from build123d import *

# Parameters (mm, degrees)
SKETCH1_R                                            = 4.5
BOSS_EXTRUDE1_DEPTH                                  = 4
SKETCH2_W                                            = 24
SKETCH2_H                                            = 6
BOSS_EXTRUDE2_DEPTH                                  = 8
CBORE_FOR_M3_HEXAGON_HEAD_BOLTS_FULL_THR_D           = 3.4
CBORE_FOR_M3_HEXAGON_HEAD_BOLTS_FULL_THR_CBORE_D     = 7
CBORE_FOR_M3_HEXAGON_HEAD_BOLTS_FULL_THR_CBORE_DEPTH = 2
FILLET1_R                                            = 10
FILLET2_R                                            = 10
SKETCH4_R                                            = 2.05
SKETCH4_R_2                                          = 1.9812
CUT_EXTRUDE2_DEPTH                                   = 51.635955605


with BuildPart() as part:
    # Sketch1 → Boss-Extrude1 (new body)
    with BuildSketch(Plane(origin=(0, 0, 0), x_dir=(1, 0, 0), z_dir=(0, 1, 0))):
        with BuildLine():
            Line((-16, 0), (-16, -30))
            Line((-16, -30), (16, -30))
            Line((16, -30), (16, 0))
            ThreePointArc((16, 0), (0, 16), (-16, 0))
        make_face()
        with Locations(Location((0, 0, 0), (0, 0, 270))):
            Circle(SKETCH1_R, mode=Mode.SUBTRACT)
    extrude(amount=BOSS_EXTRUDE1_DEPTH)

    # Sketch2 → Boss-Extrude2 (add)
    with BuildSketch(Plane(origin=(0, 4, 0), x_dir=(1, 0, 0), z_dir=(0, 1, 0))):
        with Locations((28, -3)):
            Rectangle(SKETCH2_W, SKETCH2_H)
        with Locations((-28, -3)):
            Rectangle(SKETCH2_W, SKETCH2_H)
    extrude(amount=-BOSS_EXTRUDE2_DEPTH)

    # CBORE for M3 Hexagon head bolts-Full thread-grades AB1 (through all)
    with Locations(Plane(origin=(-35, 0, 6), x_dir=(1, 0, 0), z_dir=(0, 0, 1))):
        with Locations((0, 0), (70, 0)):
            CounterBoreHole(CBORE_FOR_M3_HEXAGON_HEAD_BOLTS_FULL_THR_D / 2, CBORE_FOR_M3_HEXAGON_HEAD_BOLTS_FULL_THR_CBORE_D / 2, CBORE_FOR_M3_HEXAGON_HEAD_BOLTS_FULL_THR_CBORE_DEPTH)

    # Fillet1
    # the kernel refuses this fillet: 10 mm, written as the material it adds along each edge
    with BuildSketch(Plane(origin=(16, 0, 6), x_dir=(-1, 0, 0), z_dir=(0, 0, -1)), Plane(origin=(-16, 0, 0), x_dir=(1, 0, 0), z_dir=(0, 0, 1))) as fillet1_piece_1:
        with BuildLine():
            CenterArc((8, -10), FILLET1_R, 90, 53.130102354)
            Line((0, -4), (0, 0))
            Line((0, 0), (8, 0))
        make_face()
    extrude(amount=6)

    # Fillet2
    fillet2_edges = [part.edges().sort_by_distance(p)[0] for p in [
        (16, -4, 3),
        (-16, -4, 3),
    ]]
    fillet(fillet2_edges, radius=FILLET2_R)

    # Sketch4 → Cut-Extrude2 (cut, through all)
    # profile 1 of 4: a face of its own
    with BuildSketch(Plane(origin=(0, 4, 0), x_dir=(1, 0, 0), z_dir=(0, 1, 0))):
        with Locations(Location((-10.359727729, -15.825724364, 0), (0, 0, 270))):
            Circle(SKETCH4_R)
        with Locations((-10.359727729, -15.825724364)):
            Circle(SKETCH4_R_2, mode=Mode.SUBTRACT)
    # profile 2 of 4: a face of its own
    with BuildSketch(Plane(origin=(0, 4, 0), x_dir=(1, 0, 0), z_dir=(0, 1, 0))):
        with Locations((-10.359727729, -15.825724364)):
            Circle(SKETCH4_R_2)
    # profile 3 of 4: a face of its own
    with BuildSketch(Plane(origin=(0, 4, 0), x_dir=(1, 0, 0), z_dir=(0, 1, 0))):
        with Locations(Location((10.594689167, -15.669399213, 0), (0, 0, 270))):
            Circle(SKETCH4_R)
        with Locations((10.594689167, -15.669399213)):
            Circle(SKETCH4_R_2, mode=Mode.SUBTRACT)
    # profile 4 of 4: a face of its own
    with BuildSketch(Plane(origin=(0, 4, 0), x_dir=(1, 0, 0), z_dir=(0, 1, 0))):
        with Locations((10.594689167, -15.669399213)):
            Circle(SKETCH4_R_2)
    extrude(amount=-CUT_EXTRUDE2_DEPTH, mode=Mode.SUBTRACT)


solid = part.part
Can you work these out from the model? Positions are in its coordinate system, mm. A direction names the side the tool comes from. Coordinates: 2 decimals unless noted, no trailing zeros. Write each loop counter-clockwise with the first axis right and the second up, starting at its lowest first coordinate (ties: lowest second). Pieces come first, ordered by that corner, then holes.
Q1. Imagine slicing it at A-A, the plane x = -35. List the corners of the cut face in (y, z) for me.
Results found:
outline: (-4, 0) - (-1.7, 0) - (-1.7, 4) - (-3.5, 4) - (-3.5, 6) - (-4, 6) - close; (1.7, 0) - (4, 0) - (4, 6) - (3.5, 6) - (3.5, 4) - (1.7, 4) - close
Q2. Imagine slicing it at D-D, the plane z = 8. List the corners of the cut face in (x, y) for me, plus the area to 3 significant figures.
Results found:
outline: (-16, 0) - (16, 0) - (16, 4) - (-16, 4) - close
area: 128 mm2
Q3. Imagine slicing it at C-C, the plane y = 2.75. List the corners of the cut face in (x, z) for me, plus the area to 3 significant figures.
Results found:
outline: (-40, 0) - (-16, 0) arc R16 ccw to (16, 0) - (40, 0) - (40, 6) - (37.17, 6) - (37.17, 4) - (32.83, 4) - (32.83, 6) - (16, 6) - (16, 30) - (-16, 30) - (-16, 6) - (-32.83, 6) - (-32.83, 4) - (-37.17, 4) - (-37.17, 6) - (-40, 6) - close; hole circle Ø4.1 at (-10.36, 15.83); hole circle Ø9 at (0, 0); hole circle Ø4.1 at (10.59, 15.67)
area: 1,540 mm2
Q4. Imagine slicing it at B-B, the plane x = 0. List the corners of the cut face in (y, z) for me.
Results found:
outline: (0, -16) - (4, -16) - (4, -4.5) - (0, -4.5) - close; (0, 4.5) - (4, 4.5) - (4, 30) - (0, 30) - close
Q5. If we mould it in two halves opening along Y, with no side actions, what happens to faces 5 (the face through (32.2, -2.1, 5)), 6 (the face through (11.21, 2.028, 17.625)), 7 (the face through (-30, -4, 3)), 8 (the face through (0, 4, 5))? For each: +Y half, -Y half, draft (parallel to the pull), parting line (faces both ways), or undercut.
Results found:
face 5: undercut
face 6: draft
face 7: -Y half
face 8: +Y half
Q6. For P1, Ø16, axis at x = -5, z = 18.5, coming from the -Y side; P2, Ø2, axis at y = 2.5, z = 14, coming from the -X side; P3, Ø4, axis at x = -35, y = 0, coming from the +Z side; P4, Ø3, axis at x = -35, y = 0, coming from the -Z side, each with a flat end and sliding along its axis, tell me the tip position at first contact or that it passes through.
Results found:
P1: stops at y = 0
P2: stops at x = -16
P3: stops at z = 4
P4: passes through
Q7. Which directions (+Z, -Z, +X, -X, +Y, -Y) give clear straight access to the entire face, cutting with the end or side of a thin tool? Please do faces 1 (the face through (-38.497, 0.154, 5.014)), 2 (the face through (-16, 2, 18)), 3 (the face through (40, 0, 3)), 4 (the face through (16, 2, 18)).
Results found:
face 1: +Z
face 2: +Z, -X, +Y, -Y
face 3: +Z, -Z, +X, +Y, -Y
face 4: +Z, +X, +Y, -Y
Q8. Please list where these lines run through material, in increasing order: L1, parallel to X at y = 1.25, z = 14.5; L2, parallel to Y at x = -35, z = 1.1; L3, parallel to Y at x = -1.5, z = -10.5.
Results found:
L1: x = -16 to -11.92, -8.8 to 8.91, 12.28 to 16
L2: y = -4 to -1.7, 1.7 to 4
L3: y = 0 to 4
